For this review, take the finished solid that the model builds, in its own axes (mm). Face numbers are marked on the shaded views. A direction names the side the tool comes from. Coordinates: 2 decimals unless noted, no trailing zeros. Loops run counter-clockwise (first coordinate to the right, second up) from the corner with the lowest first, then second, coordinate; pieces in that order, holes last. Notation, with made-up numbers: (10.5, 7) -> (51.5, 7) arc R25 cw to (51.5, 34) -> close; hole circle Ø3 at (65, -24.75). An arc over 180 degrees is marked (long way). One line per item, written item: value.
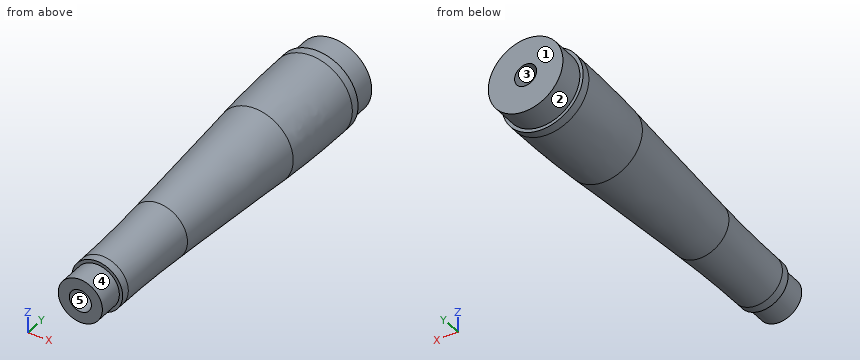
from build123d import *


# Not quite as in the source:
# - a fillet or chamfer that OpenCascade refuses, or shapes differently, is made with other operations: its cross-section is extruded or revolved along the edge and cut away or added


with BuildPart() as f1:
    # F0 (on Top) → F1 (revolve)
    with BuildSketch(Plane.XY):
        Polygon((14.7, 0), (4.35, 0), (4.35, -12), (9.35, -17), (6.35, -136), (4.35, -138), (4.35, -150), (8.7, -150), (8.7, -140), (10, -140), (10, -120), (16, -30), (16, -10), (14.7, -10), align=None)
    revolve(axis=Axis((0, -75, 0), (0, 1, 0)))

    # F2: fillet of radius 500 on 2 edges, made by hand

    # F2_s1 → F2_t2 (revolve, cut)
    with BuildSketch(Plane.XY):
        with BuildLine():
            ThreePointArc((14.8925789283, -46.6113160754), (15.7230680408, -29.9907791687), (16, -13.3518108135))
            Line((16, -13.3518108135), (16, -30))
            Line((16, -30), (14.8925789283, -46.6113160754))
        make_face()
    revolve(axis=Axis((0, -30, 0), (0, 1, 0)), mode=Mode.SUBTRACT)

    # F2_s3 → F2_t4 (revolve)
    with BuildSketch(Plane.XY):
        with BuildLine():
            ThreePointArc((11.1074210717, -103.3886839246), (10.2769319592, -120.0092208313), (10, -136.6481891865))
            Line((10, -136.6481891865), (10, -120))
            Line((10, -120), (11.1074210717, -103.3886839246))
        make_face()
    revolve(axis=Axis((0, -120, 0), (0, 1, 0)))


solid = f1.part
1. Take a section at B-B, the plane y = -49. Give the boundary of the cut face in (x, z).
Return value:
outline: circle Ø29.47 at (0, 0); hole circle Ø17.09 at (0, 0)
2. For the marked faces 4 and 5, list the 3-axis set-ups (+Z, -Z, +X, -X, +Y, -Y) from which the entire face can be reached by the end or side of a thin tool; tool diameter is ignored.
Return value:
face 4: -Y
face 5: +Y, -Y
3. The part is to be moulded in two halves that separate along Z. For the marked faces 1, 2 and 3, say which applies: pulls with the +Z half, pulls with the -Z half, needs draft (parallel to the pull), parting line crosses it, or undercut.
Return value:
face 1: needs draft
face 2: parting line crosses it
face 3: undercut
4. Insertion check: pin 1 Ø2 at (y, z) = (-133.5, -12.5) entering from -X; pin 2 Ø8 at (y, z) = (-65, -3) entering from -X; pin 3 Ø2 at (x, y) = (-11, -36.5) entering from -Z; pin 4 Ø6 at (y, z) = (-34.5, 11) entering from -X. Each pin has a flat end and moves straight along its axis. Give the tip position at first contact, or say it passes through.
Return value:
pin 1: passes through
pin 2: stops at x = -13.87
pin 3: stops at z = -11.8
pin 4: stops at x = -13.34
5. Take a section at A-A, the plane y = -73. Give the boundary of the cut face in (x, z), and give its area (3 significant figures).
Return value:
outline: circle Ø26.27 at (0, 0); hole circle Ø15.88 at (0, 0)
area: 344 mm2
6. To check wall thickness, follow probe 1 along Z at (x, y) = (0, -145.25); probe 2 along Z at (x, y) = (0, -4.75). State the ranges of each line that lie inside material, in increasing order. Write a range as from..to.
Return value:
probe 1: z = -8.7..-4.35, 4.35..8.7
probe 2: z = -14.7..-4.35, 4.35..14.7
